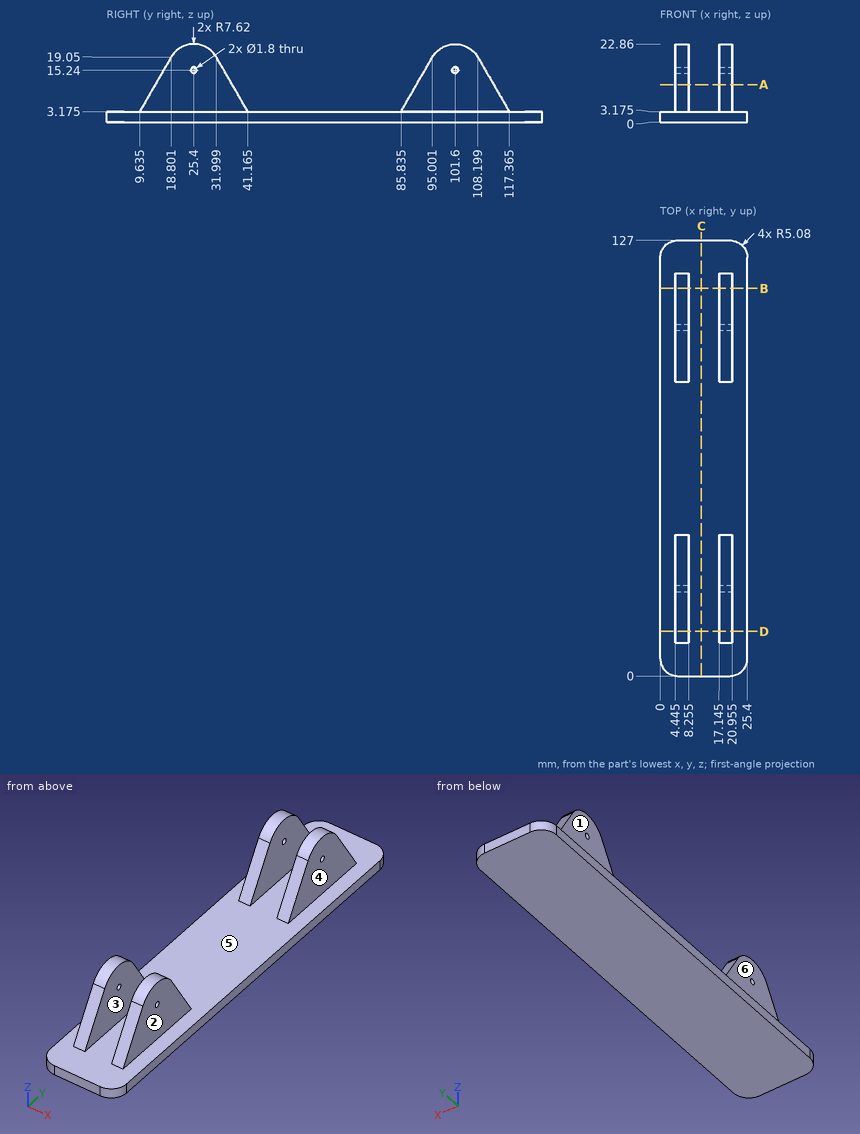
Verification items for this drawing (mm, ordinates from the low corner). A direction names the side the tool comes from. Coordinates: 2 decimals unless noted, no trailing zeros. Loops run counter-clockwise (first coordinate to the right, second up) from the corner with the lowest first, then second, coordinate; pieces in that order, holes last. Notation, with made-up numbers: (-29.75, 3.25) -> (-10.75, 3.25) arc R12 ccw to (-10.75, 12.25) -> close; hole circle Ø5 at (85, -5.75). An arc over 180 degrees is marked (long way). Put each result on its own line as item: value.
1. Tool access check on the marked faces 1, 2 and 3. Record the directions out of +Z, -Z, +X, -X, +Y, -Y that give a thin tool (end or side, any length) a straight path to the whole face; none if there is none.
Result set:
face 1: +Z, -X, +Y, -Y
face 2: +Z, +X, +Y, -Y
face 3: +Z, +Y, -Y
2. Mould release check, pull along X, two halves, no side actions. Record for the marked faces 4, 5 and 6: pulls with the +X half, pulls with the -X half, needs draft (parallel to the pull), parting line crosses it, or undercut.
Result set:
face 4: pulls with the +X half
face 5: undercut
face 6: pulls with the -X half
3. Section check A-A, the plane z = 11. Record the boundary of the cut face in (x, y) (1 decimal).
Result set:
outline: (4.4, 14.2) -> (8.3, 14.2) -> (8.3, 36.6) -> (4.4, 36.6) -> close; (4.4, 90.4) -> (8.3, 90.4) -> (8.3, 112.8) -> (4.4, 112.8) -> close; (17.1, 14.2) -> (21, 14.2) -> (21, 36.6) -> (17.1, 36.6) -> close; (17.1, 90.4) -> (21, 90.4) -> (21, 112.8) -> (17.1, 112.8) -> close
4. Gauge pin test, flat ends, axial feed: P1, Ø2, axis at y = 101.6, z = 15.24, coming from the +X side (3 decimals); P2, Ø6, axis at y = 24, z = 11.5, coming from the -X side (3 decimals); P3, Ø7.5, axis at x = 9.5, y = 71.5, coming from the +Z side (3 decimals). Record the tip position at first contact, or that the pin passes through.
Result set:
P1: stops at x = 20.955
P2: stops at x = 4.445
P3: stops at z = 3.175
5. Section check C-C, the plane x = 12. Record the boundary of the cut face in (y, z) (1 decimal).
Result set:
outline: (0, 0) -> (127, 0) -> (127, 3.2) -> (0, 3.2) -> close
6. Thickness scan on line 1 (Z direction, x = 20.15, y = 101.6); line 2 (X direction, y = 38, z = 4.25) (1 decimal); line 3 (Y direction, x = 20, z = 14.5) (1 decimal). Record the ranges inside material, lowest first.
Result set:
line 1: z = 0 to 14.34, 16.14 to 22.86
line 2: x = 4.4 to 8.3, 17.1 to 21
line 3: y = 16.2 to 24.9, 25.9 to 34.6, 92.4 to 101.1, 102.1 to 110.8
7. Section check B-B, the plane y = 113. Record the boundary of the cut face in (x, z) (1 decimal).
Result set:
outline: (0, 0) -> (25.4, 0) -> (25.4, 3.2) -> (21, 3.2) -> (21, 10.7) -> (17.1, 10.7) -> (17.1, 3.2) -> (8.3, 3.2) -> (8.3, 10.7) -> (4.4, 10.7) -> (4.4, 3.2) -> (0, 3.2) -> close
8. Section check D-D, the plane y = 13. Record the boundary of the cut face in (x, z) (1 decimal).
Result set:
outline: (0, 0) -> (25.4, 0) -> (25.4, 3.2) -> (21, 3.2) -> (21, 9) -> (17.1, 9) -> (17.1, 3.2) -> (8.3, 3.2) -> (8.3, 9) -> (4.4, 9) -> (4.4, 3.2) -> (0, 3.2) -> close
